CAD build for the part. Positions are in the model's coordinates, mm. A direction names the side the tool comes from. Give positions to 0.01 mm unless a question says otherwise; leave off trailing zeros. Order: outer loops, then holes, each group sorted by start corner. A loop starts at its lowest first (then second) coordinate and runs counter-clockwise, first axis right, second up.
Item 1: Band-saw the part on A-A on z = 4. Give the cut face in (x, y).
Item 2: Which spindle directions (+Z, -Z, +X, -X, +Y, -Y) get a long thin tool onto all of the face, cutting with end or side? Do faces 4 (the flat face through (9, 26, -6)), 5 (the flat face through (-32, 3, 8)), 6 (the flat face through (-32, 10, -2)). Say none if no direction does.
Item 3: Band-saw the part on C-C on x = -1.5. Give the cut face in (y, z), plus the area to 3 significant figures.
Item 4: Two-plate mould, pull along Z, no slides. Class faces 1 (the flat face through (-17, 6, 14)), 2 (the flat face through (9, 26, 6)), 3 (the flat face through (0, 30, 10)): released by +Z, released by -Z, zero draft, split by the parting line, or undercut.
Item 5: Wall check: L1, parallel to Z at x = 0, y = 10.25; L2, parallel to Y at x = -27, z = -7. Give the ranges that are in metal, low to high.
Item 6: Band-saw the part on B-B on y = 27.25. Give the cut face in (x, z).
Item 7: Band-saw the part on D-D on y = 7.75. Give the cut face in (x, z).
Item 8: Flat gauge pins, fed straight in: P1, Ø1.5, axis at y = 6, z = 5, coming from the -X side; P2, Ø6, axis at x = -10.5, y = 24, coming from the +Z side; P3, Ø13, axis at x = -28.5, z = 2, coming from the +Y side. Where does each tip first touch, or does it go through?
Autodesk Inventor part; units mm, degrees
ref_plane "YZ Plane" through (0, 0, 0) normal (1, 0, 0) x (0, 1, 0)
ref_plane "XZ Plane" through (0, 0, 0) normal (0, 1, 0) x (-1, 0, 0)
ref_plane "XY Plane" through (0, 0, 0) normal (0, 0, 1) x (1, 0, 0)
sketch "草图1" plane through (0, 0, 0) normal (0, 1, 0) x (-1, 0, 0)
  circle A0 centre (0, 0) radius 8
  circle A1 centre (0, 0) radius 14
  dimension "d0" = 16
  dimension "d1" = 28
extrude "拉伸1" add sketch "草图1" along normal blind 30
sketch "草图2" plane through (0, 30, 0) normal (0, 1, 0) x (1, 0, 0)
  circle A0 centre (0, 0) radius 14
  line L0 (18.1173, -6) -> (-18.1173, -6)
  line L1 (-18.1173, -6) -> (-18.1173, 6)
  line L2 (-18.1173, 6) -> (18.1173, 6)
  line L3 (18.1173, 6) -> (18.1173, -6)
  line L4 (18.1173, -6) -> (-18.1173, 6) construction
  line L5 (-18.1173, -6) -> (18.1173, 6) construction
  dimension "d4" = 12
  dimension "d5" = 36.2346
extrude "拉伸2" cut sketch "草图2" against normal blind 9 contours A0 L0 L2 | A0 L2 L3 L0 | A0 L0 L1 L2
sketch "草图3" plane through (0, 0, 0) normal (0, -1, 0) x (1, 0, 0)
  circle A0 centre (0, 0) radius 14
  line L0 (0, 14) -> (-35, 14)
  line L1 (0, -14) -> (-35, -14)
  line L2 (-41.9506, 4) -> (-20.5959, 4)
  arc A1 (-29, 0) -> (-29, 8) centre (-29, 4) ccw
  line L3 (-29, 8) -> (-35, 8)
  line L4 (-29, 0) -> (-35, 0)
  line L5 (-35, 14) -> (-35, 8)
  line L6 (-35, 0) -> (-35, -14)
  dimension "d8" = 8
  dimension "d9" = 35
  dimension "d10" = 35
  dimension "d11" = 6
  dimension "d12" = 6
sketch "草图4" plane through (0, 0, 0) normal (0, -1, 0) x (1, 0, 0)
  circle A0 centre (0, 0) radius 8
  circle A1 centre (0, 0) radius 14
extrude "拉伸3" add sketch "草图3" against normal blind 12 contours A0 L1 L6 L4 A1 L3 L5 L0
sketch "草图5" plane through (0, 12, 0) normal (0, 1, 0) x (1, 0, 0)
  line L0 (-35, 14) -> (-35, 0)
  line L1 (-35, 0) -> (-29, 0)
  arc A0 (-29, -8) -> (-29, 0) centre (-29, -4) ccw
  line L2 (-29, -8) -> (-35, -8)
  line L3 (-35, -8) -> (-35, -14)
  arc A1 (-29, -10) -> (-29, 2) centre (-29, -4) ccw
  line L4 (-29, 2) -> (-35, 2)
  line L5 (-29, -10) -> (-35, -10)
  dimension "d15" = 12
extrude "拉伸4" cut sketch "草图5" against normal blind 5
The answers:
1. outline: (-25, 0) - (-6.93, 0) - (-6.93, 21) - (-13.42, 21) - (-13.42, 12) - (-23, 12) - (-23, 7) - (-25, 7) - close; (6.93, 0) - (13.42, 0) - (13.42, 21) - (6.93, 21) - close
2. face 4: +X, -X, +Y
2. face 5: -X, +Y, -Y
2. face 6: -X, +Y
3. outline: (0, -14) - (12, -14) - (12, -13.92) - (30, -13.92) - (30, -7.86) - (0, -7.86) - close; (0, 7.86) - (30, 7.86) - (30, 13.92) - (12, 13.92) - (12, 14) - (0, 14) - close
3. area: 366 mm2
4. face 1: released by +Z
4. face 2: undercut
4. face 3: zero draft
5. L1: z = -14 to -8, 8 to 14
5. L2: y = 0 to 12
6. outline: (-12.65, -6) arc R14 ccw to (12.65, -6) - (5.29, -6) arc R8 cw to (-5.29, -6) - close; (-12.65, 6) - (-5.29, 6) arc R8 cw to (5.29, 6) - (12.65, 6) arc R14 ccw to start
7. outline: (-35, -14) - (0, -14) arc R14 ccw to (0, 14) - (-35, 14) - (-35, 10) - (-29, 10) arc R6 cw to (-29, -2) - (-35, -2) - close; hole circle Ø16 at (0, 0)
8. P1: stops at x = -25.4
8. P2: stops at z = 11.82
8. P3: stops at y = 12
